from build123d import *

# Parameters (mm, degrees)
SKETCH006_R             = 10.24367
SKETCH006_R_2           = 1.237403
PAD005_DEPTH            = 5.8
PAD006_DEPTH            = 1
SKETCH008_R             = 7.5076691177
PAD007_DEPTH            = 5
SKETCH009_W             = 33.111977
SKETCH009_H             = 4.462531
POCKET001_DEPTH         = 9
BODY001_PLACEMENT_ANGLE = 90


with BuildPart() as part:
    # Sketch006 → Pad005 (new body)
    with BuildSketch(Plane.XY):
        with BuildLine():
            Line((-18.4256, -1.34093), (-18.409945, -21.590897))
            Line((-18.409945, -21.590897), (16.494272, -21.597601))
            Line((16.494272, -21.597601), (16.2785, -4.27596))
            add(Edge.make_bspline(
                [(-18.4256, -1.34093), (-17.942909, 6.597493), (-8.092874, 14.805856), (3.694337, 13.295516), (9.670027, 9.683837), (13.4539, 4.00771), (16.2785, -4.27596)],
                knots=[0, 0, 0, 0, 0.25, 0.5, 0.75, 1, 1, 1, 1], degree=3))
        make_face()
        with Locations((-3.602271, -3.847481)):
            Circle(SKETCH006_R, mode=Mode.SUBTRACT)
        with Locations((-16.625307, -18.983036)):
            Circle(SKETCH006_R_2, mode=Mode.SUBTRACT)
    extrude(amount=PAD005_DEPTH)

    # Sketch007 → Pad006 (join)
    with BuildSketch(Plane.XY):
        Polygon((-8.077186, 5.935153), (-7.114697, 3.787175), (-10.68287, -7.783438), (-12.927779, -9.78625), (-8.900146, -13.417724), (-6.14903, -9.720223), (0.343604, -8.795849), (5.141551, -10.468527), (6.924273, -6.550939), (2.544497, -5.208394), (-3.520839, 4.178236), (-4.27353, 7.000822), align=None)
    extrude(amount=PAD006_DEPTH)

    # Sketch008 → Pad007 (join)
    with BuildSketch(Plane.XY):
        with Locations((-4.582225, -3.257763)):
            Circle(SKETCH008_R)
    extrude(amount=PAD007_DEPTH)

    # Sketch009 (on Face3 of Pad007) → Pocket001 (cut)
    with BuildSketch(Plane(origin=(-0.0041476098, -21.5944321736, 0), x_dir=(0.9999999816, -0.0001920685, 0), z_dir=(-0.0001920685, -0.9999999816, 0))):
        with Locations((-0.9438935, 2.7535015)):
            Rectangle(SKETCH009_W, SKETCH009_H)
    extrude(amount=-POCKET001_DEPTH, mode=Mode.SUBTRACT)


with BuildPart() as part_1:
    # Body001 placement: moved
    add(part.part.moved(Location((-47, -2.9, 4))).rotate(Axis((-47, -2.9, 4), (0, 0, 1)), BODY001_PLACEMENT_ANGLE))


solid = part_1.part
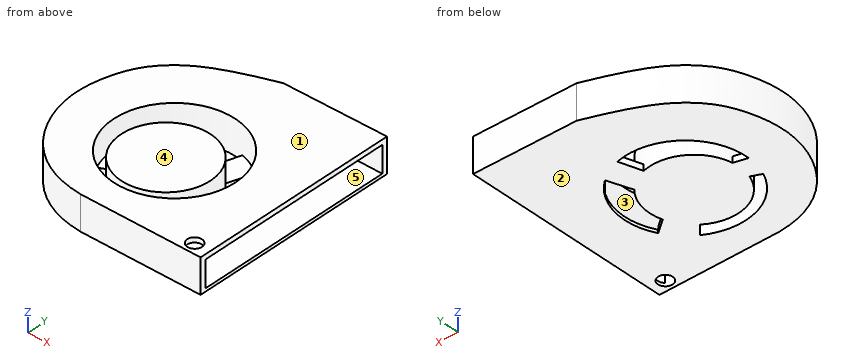
The listing builds one solid part. Answer for the finished solid, in the listing's coordinates (mm). Face numbers are marked on the shaded views. A direction names the side the tool comes from. Coordinates: 2 decimals unless noted, no trailing zeros. Write each loop counter-clockwise with the first axis right and the second up, starting at its lowest first coordinate (ties: lowest second). Pieces come first, ordered by that corner, then holes. Notation, with made-up numbers: (77.25, 80) - (131.25, 80) arc R24 cw to (131.25, 109) - close; hole circle Ø7 at (17, 45.25). An arc over 180 degrees is marked (long way). Put each result on its own line as item: value.
1. Find the intervals of material crossed by line 1 along Z through (x, y) = (-30, -17); line 2 along Y through (x, z) = (-45.5, 8.85); line 3 along Y through (x, z) = (-44, 5.5), in increasing order. Write a range as from..to.
Answer sheet:
line 1: z = 4..4.52, 8.98..9.8
line 2: y = -21.33..-16.47, -14.78..-0.18, 3.47..12.39
line 3: y = -21.32..-16.71, -14.99..0.02, 3.71..12.94
2. The part is cut by section A-A on x = -35. Give the vertices of the cut face in (y, z), plus the area to 3 significant figures.
Answer sheet:
outline: (-21.32, 4) - (-10.75, 4) - (-10.75, 5) - (-12.7, 5) - (-12.7, 9.8) - (-21.32, 9.8) - close; (-0.3, 4) - (13.47, 4) - (13.47, 9.8) - (-0.3, 9.8) - close
area: 132 mm^2
3. A tool of negligible diameter and unlimited length cuts with its end or side. For the marked faces 4 and 5, from which of +Z, -Z, +X, -X, +Y, -Y can it reach the whole face along a straight path? Write none if from no direction.
Answer sheet:
face 4: +Z
face 5: +X
4. The part is cut by section B-B on y = -4.5. State how many separate pieces and enclosed holes the cut face has, plus the area to 3 significant figures.
Answer sheet:
separate pieces: 4
enclosed holes: 0
area: 123 mm^2
5. Determine the mould class of the marked faces 1, 2 and 3 for opening direction Z: pulls with the +Z half, pulls with the -Z half, needs draft (parallel to the pull), parting line crosses it, or undercut.
Answer sheet:
face 1: pulls with the +Z half
face 2: pulls with the -Z half
face 3: undercut
6. The part is cut by section C-C on x = -40. Give the vertices of the cut face in (y, z), plus the area to 3 significant figures.
Answer sheet:
outline: (-21.32, 4) - (-16.25, 4) - (-16.25, 9.8) - (-21.32, 9.8) - close; (-13.99, 4) - (13.41, 4) - (13.41, 9.8) - (3.24, 9.8) - (3.24, 5) - (-0.97, 5) - (-0.97, 9) - (-13.99, 9) - close
area: 158 mm^2
7. Flat-ended cylindrical pins translate along their axes: pin 1 Ø1.3 at (x, z) = (-28.5, 6.5) entering from -Y; pin 2 Ø1.3 at (x, z) = (-30.5, 6.5) entering from +Y; pin 3 Ø2 at (y, z) = (6.5, 7.5) entering from +X. Find the tip coordinate at first contact, or state that the pin passes through.
Answer sheet:
pin 1: stops at y = -21.31
pin 2: stops at y = 13.54
pin 3: stops at x = -34.4
